from build123d import *

# Parameters (mm, degrees)
F1_DEPTH = 25.4
F2_R     = 21.201503
F3_DEPTH = 25.401
F4_R     = 12.7
F5_R     = 12.7
F6_R     = 12.7
F7_R     = 12.7
F8_R     = 21.507739
F9_DEPTH = 25.401


with BuildPart() as f1:
    # F0 (on Top) → F1 (new body)
    with BuildSketch(Plane.XY):
        with BuildLine():
            ThreePointArc((24.118333, -0.702734), (13.366391, 34.203378), (-20.838827, 47.011342))
            ThreePointArc((-20.838827, 47.011342), (-85.141829, 72.076017), (-58.070359, 8.591772))
            ThreePointArc((-58.070359, 8.591772), (-42.025812, -26.985416), (-3.531117, -33.413651))
            ThreePointArc((-3.531117, -33.413651), (62.977366, -61.590022), (24.118333, -0.702734))
        make_face()
    extrude(amount=F1_DEPTH)

    # F2 (on face) → F3 (cut, through all)
    with BuildSketch(Plane.XY.offset(25.4)):
        with Locations((-58.259711, 46.025168)):
            Circle(F2_R)
    extrude(amount=-F3_DEPTH, mode=Mode.SUBTRACT)

    # F4
    f4_edges = [f1.edges().sort_by_distance(p)[0] for p in [
        (-3.531117, -33.413651, 12.7),
    ]]
    fillet(f4_edges, radius=F4_R)

    # F5
    f5_edges = [f1.edges().sort_by_distance(p)[0] for p in [
        (24.118333, -0.702734, 12.7),
    ]]
    fillet(f5_edges, radius=F5_R)

    # F6
    f6_edges = [f1.edges().sort_by_distance(p)[0] for p in [
        (-20.838827, 47.011342, 12.7),
    ]]
    fillet(f6_edges, radius=F6_R)

    # F7
    f7_edges = [f1.edges().sort_by_distance(p)[0] for p in [
        (-58.070359, 8.591772, 12.7),
    ]]
    fillet(f7_edges, radius=F7_R)

    # F8 (on face) → F9 (cut, through all)
    with BuildSketch(Plane.XY.offset(25.4)):
        with Locations((34.096744, -37.178192)):
            Circle(F8_R)
    extrude(amount=-F9_DEPTH, mode=Mode.SUBTRACT)


solid = f1.part
Could you check a few things on this model? Use its own coordinates, in mm. Round coordinates to 2 decimals unless told otherwise and drop trailing zeros. Write each loop counter-clockwise with the first axis right and the second up, starting at its lowest first coordinate (ties: lowest second). Pieces come first, ordered by that corner, then holes. Notation, with made-up numbers: (70.25, 8) -> (114.25, 8) arc R27 cw to (114.25, 45) -> close; hole circle Ø6 at (32, -20.5). An arc over 180 degrees is marked (long way). Use a Markdown table: item, result.
1. If we section it at A-A (y = 41): List the corners of the cut face in (x, z) for me.
Answer key:
| item | result |
|---|---|
| outline | (-95.35, 0) -> (-78.86, 0) -> (-78.86, 25.4) -> (-95.35, 25.4) -> close; (-37.66, 0) -> (5.05, 0) -> (5.05, 25.4) -> (-37.66, 25.4) -> close |
2. We'd pull the mould along X, two halves only. Please class faces 1 (the face through (62.205, -62.475, 12.522)), 2 (the face through (-79.44, 46.96, 12.88)), 3 (the face through (53.964, -45.416, 12.878)), 4 (the face through (12.598, 34.997, 12.522)): +X half, -X half, draft (parallel to the pull), parting line (faces both ways), or undercut.
Answer key:
| item | result |
|---|---|
| face 1 | parting line |
| face 2 | undercut |
| face 3 | undercut |
| face 4 | +X half |
3. For pin 1 Ø6 at (x, z) = (41.5, 12) entering from +Y; pin 2 Ø2 at (y, z) = (48, 18.5) entering from -X; pin 3 Ø5 at (y, z) = (4, 21.5) entering from -X, each with a flat end and sliding along its axis, tell me the tip position at first contact or that it passes through.
Answer key:
| item | result |
|---|---|
| pin 1 | stops at y = 0.38 |
| pin 2 | stops at x = -95.68 |
| pin 3 | stops at x = -61.41 |
4. If we section it at D-D (x = -85): List the corners of the cut face in (y, z) for me.
Answer key:
| item | result |
|---|---|
| outline | (19.83, 0) -> (72.22, 0) -> (72.22, 25.4) -> (19.83, 25.4) -> close |
5. Please list where these lines run through material, in increasing order: probe 1 along Y at (x, z) = (-75, 14); probe 2 along X at (y, z) = (39.5, 16.75); probe 3 along Y at (x, z) = (-66.5, 3.5).
Answer key:
| item | result |
|---|---|
| probe 1 | y = 12.54 to 33.01, 59.04 to 79.51 |
| probe 2 | x = -95.12 to -78.43, -38.09 to 7.3 |
| probe 3 | y = 9.48 to 26.49, 65.56 to 82.54 |
6. If we section it at B-B (x = 18): List the corners of the cut face in (y, z) for me.
Answer key:
| item | result |
|---|---|
| outline | (-71.4, 0) -> (-51.44, 0) -> (-51.44, 25.4) -> (-71.4, 25.4) -> close; (-22.91, 0) -> (28.29, 0) -> (28.29, 25.4) -> (-22.91, 25.4) -> close |
7. If we section it at C-C (z = 4): State how many separate pieces and enclosed holes the cut face has, then the cut area to 3 significant figures.
Answer key:
| item | result |
|---|---|
| separate pieces | 1 |
| enclosed holes | 2 |
| area | 10,400 mm^2 |
